from build123d import *

# Parameters (mm, degrees)
CROQUIS1_W              = 45
CROQUIS1_H              = 21
CROQUIS1_R              = 0.625
SALIENTE_EXTRUIR1_DEPTH = 1.5
CROQUIS2_R              = 8
SALIENTE_EXTRUIR2_DEPTH = 10


with BuildPart() as part:
    # Croquis1 → Saliente-Extruir1 (new body)
    with BuildSketch(Plane.XY):
        with Locations((22.5, 10.5)):
            Rectangle(CROQUIS1_W, CROQUIS1_H)
        with Locations((1.425, 19.575)):
            Circle(CROQUIS1_R, mode=Mode.SUBTRACT)
        with Locations(Location((43.575, 19.575, 0), (0, 0, 180))):
            Circle(CROQUIS1_R, mode=Mode.SUBTRACT)
        with Locations((43.575, 1.425)):
            Circle(CROQUIS1_R, mode=Mode.SUBTRACT)
        with Locations(Location((1.425, 1.425, 0), (0, 0, 180))):
            Circle(CROQUIS1_R, mode=Mode.SUBTRACT)
    extrude(amount=SALIENTE_EXTRUIR1_DEPTH)

    # Croquis2 → Saliente-Extruir2 (add)
    with BuildSketch(Plane(origin=(0, 0, 0), x_dir=(-1, 0, 0), z_dir=(0, 0, -1))):
        with Locations((-35, 10.5)):
            Circle(CROQUIS2_R)
        with Locations(Location((-10, 10.5, 0), (0, 0, 180))):
            Circle(CROQUIS2_R)
    extrude(amount=SALIENTE_EXTRUIR2_DEPTH)


solid = part.part
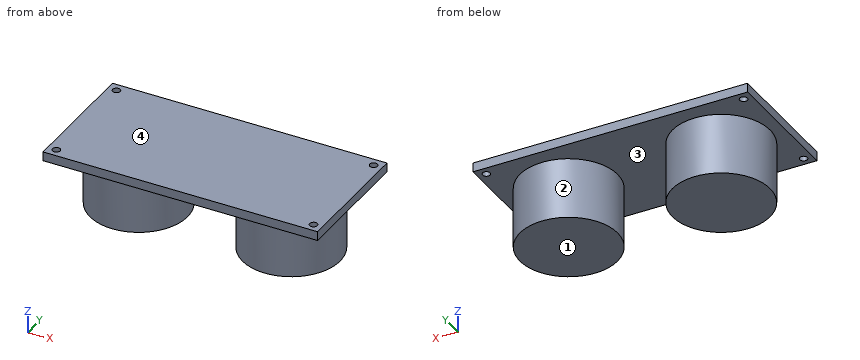
Geometry check sheet. Reference: the model listing, model coordinates, mm. Face numbers are marked on the shaded views. A direction names the side the tool comes from. Round coordinates to 2 decimals unless told otherwise and drop trailing zeros. Order: outer loops, then holes, each group sorted by start corner. A loop starts at its lowest first (then second) coordinate and runs counter-clockwise, first axis right, second up. Notation, with made-up numbers: (18.5, 56.25) - (44.5, 56.25) arc R19 cw to (44.5, 66.25) - close; hole circle Ø9 at (-12, 82). An arc over 180 degrees is marked (long way). One line per question, with ' | ' between items. Start each with the question number.
(1) Sectioned sample at B-B on z = -5.5. Record the cut outline in (x, y), and give its area (3 significant figures).
(2) Sectioned sample at A-A on y = 10.5. Record the cut outline in (x, z), and give its area (4 significant figures).
(3) Access from +Z, -Z, +X, -X, +Y, -Y to the whole of each face (thin tool, end or side, straight path). Record for the marked faces 1 and 2.
(4) Depth check by flat-ended pin: pin 1 Ø2 at (x, y) = (1.425, 1.425) entering from -Z; pin 2 Ø1.5 at (x, z) = (8.5, -2.5) entering from -Y; pin 3 Ø2 at (y, z) = (15, -4.5) entering from -X; pin 4 Ø0.8 at (x, y) = (43.575, 1.425) entering from -Z. Enter the tip coordinate at first touch or a pass-through.
(5) Thickness scan on L1, parallel to X at y = 10.25, z = -3.75; L2, parallel to Z at x = 6, y = 19; L3, parallel to X at y = 12.25, z = -5.25. Record the ranges inside material, lowest first. Write a range as [from, to].
(6) Sectioned sample at C-C on x = 10. Record the cut outline in (y, z).
(7) Sectioned sample at D-D on x = 39.5. Record the cut outline in (y, z).
(8) Release check for a two-part mould opening along X. For the marked faces 3 and 4 record: released by +X, released by -X, zero draft, split by the parting line, or undercut.
Conclusion:
1) outline: circle Ø16 at (10, 10.5); circle Ø16 at (35, 10.5) | area: 402 mm2
2) outline: (0, 0) - (2, 0) - (2, -10) - (18, -10) - (18, 0) - (27, 0) - (27, -10) - (43, -10) - (43, 0) - (45, 0) - (45, 1.5) - (0, 1.5) - close | area: 387.5 mm2
3) face 1: -Z, +X, -X, +Y, -Y | face 2: -Z
4) pin 1: stops at z = 0 | pin 2: stops at y = 2.54 | pin 3: stops at x = 2.81 | pin 4: passes through
5) L1: x = [2, 18], [27, 43] | L2: z = [0, 1.5] | L3: x = [2.19, 17.81], [27.19, 42.81]
6) outline: (0, 0) - (2.5, 0) - (2.5, -10) - (18.5, -10) - (18.5, 0) - (21, 0) - (21, 1.5) - (0, 1.5) - close
7) outline: (0, 0) - (3.89, 0) - (3.89, -10) - (17.11, -10) - (17.11, 0) - (21, 0) - (21, 1.5) - (0, 1.5) - close
8) face 3: undercut | face 4: zero draft
